```python
from build123d import *

# Parameters (mm, degrees)
SKETCH1_W           = 98
SKETCH1_H           = 98
BOSS_EXTRUDE1_DEPTH = 40
SKETCH2_W           = 94
SKETCH2_H           = 94
CUT_EXTRUDE1_DEPTH  = 5
SKETCH3_W           = 90
SKETCH3_H           = 90
CUT_EXTRUDE2_DEPTH  = 30
SKETCH4_W           = 98
SKETCH4_H           = 98
SKETCH4_W_2         = 94
SKETCH4_H_2         = 94
CUT_EXTRUDE3_DEPTH  = 1.8
SKETCH5_R           = 1.3
BOSS_EXTRUDE2_DEPTH = 2.5
FILLET1_R           = 1.5
FILLET2_R           = 1.5


with BuildPart() as part:
    # Sketch1 → Boss-Extrude1 (new body)
    with BuildSketch(Plane(origin=(0, 0, 0), x_dir=(1, 0, 0), z_dir=(0, 1, 0))):
        Rectangle(SKETCH1_W, SKETCH1_H)
    extrude(amount=BOSS_EXTRUDE1_DEPTH)

    # Sketch2 → Cut-Extrude1 (cut)
    with BuildSketch(Plane(origin=(0, 40, 0), x_dir=(1, 0, 0), z_dir=(0, 1, 0))):
        Rectangle(SKETCH2_W, SKETCH2_H)
    extrude(amount=-CUT_EXTRUDE1_DEPTH, mode=Mode.SUBTRACT)

    # Sketch3 → Cut-Extrude2 (cut)
    with BuildSketch(Plane(origin=(0, 35, 0), x_dir=(1, 0, 0), z_dir=(0, 1, 0))):
        Rectangle(SKETCH3_W, SKETCH3_H)
    extrude(amount=-CUT_EXTRUDE2_DEPTH, mode=Mode.SUBTRACT)

    # Sketch4 → Cut-Extrude3 (cut)
    with BuildSketch(Plane(origin=(0, 40, 0), x_dir=(1, 0, 0), z_dir=(0, 1, 0))):
        Rectangle(SKETCH4_W, SKETCH4_H)
        Rectangle(SKETCH4_W_2, SKETCH4_H_2, mode=Mode.SUBTRACT)
    extrude(amount=-CUT_EXTRUDE3_DEPTH, mode=Mode.SUBTRACT)

    # Sketch5 → Boss-Extrude2 (add)
    with BuildSketch(Plane(origin=(0, 38.2, 0), x_dir=(1, 0, 0), z_dir=(0, 1, 0))):
        with BuildLine():
            Line((-49, 4), (-51, 4))
            ThreePointArc((-51, 4), (-55, 0), (-51, -4))
            Line((-51, -4), (-49, -4))
            Line((-49, -4), (-49, 4))
        make_face()
        with Locations((-52.4, 0)):
            Circle(SKETCH5_R, mode=Mode.SUBTRACT)
        with BuildLine():
            Line((49, 4), (49, -4))
            Line((49, -4), (51, -4))
            ThreePointArc((51, -4), (55, 0), (51, 4))
            Line((51, 4), (49, 4))
        make_face()
        with Locations((52.4, 0)):
            Circle(SKETCH5_R, mode=Mode.SUBTRACT)
    extrude(amount=-BOSS_EXTRUDE2_DEPTH)

    # Fillet1
    fillet1_edges = [part.edges().sort_by_distance(p)[0] for p in [
        (-49, 35.7, 0),
        (-49, 36.95, -4),
        (-49, 36.95, 4),
    ]]
    fillet(fillet1_edges, radius=FILLET1_R)

    # Fillet2
    fillet2_edges = [part.edges().sort_by_distance(p)[0] for p in [
        (49, 36.95, -4),
        (49, 35.7, 0),
        (49, 36.95, 4),
    ]]
    fillet(fillet2_edges, radius=FILLET2_R)


solid = part.part
```
Part model, mm, in its own coordinate system. A direction names the side the tool comes from. Coordinates: 2 decimals unless noted, no trailing zeros. Order: outer loops, then holes, each group sorted by start corner. A loop starts at its lowest first (then second) coordinate and runs counter-clockwise, first axis right, second up. Notation, with made-up numbers: (23.5, -6) - (43.5, -6) arc R27 ccw to (43.5, 21) - close; hole circle Ø6 at (81.5, 40.5). An arc over 180 degrees is marked (long way). Return JSON: item names as keys, results as strings. Group by question number.
Item 1: Cut at D-D (z = 43). List the corners of the cut face in (x, y), plus the area to 3 significant figures.
Item 2: Which spindle directions (+Z, -Z, +X, -X, +Y, -Y) get a long thin tool onto all of the face, cutting with end or side? Do faces 1 (the face through (-1, 37, -47)), 2 (the face through (-54, 35.7, 0)), 3 (the face through (54, 35.7, 0)). Say none if no direction does.
Item 3: Cut at B-B (y = 9.5). List the corners of the cut face in (x, z), plus the area to 3 significant figures.
Item 4: Cut at A-A (z = 0). List the corners of the cut face in (x, y).
Item 5: Pin check, flat tips, straight feed: pin 1 (8 mm diameter, centred on x = -2, z = 19.5, fed in from +Y); pin 2 (1 mm diameter, centred on y = 37, z = 11.5, fed in from +X); pin 3 (1 mm diameter, centred on y = 36.5, z = -6.5, fed in from -X); pin 4 (1.3 mm diameter, centred on x = -52, z = 0, fed in from -Y). Stop position of each tip, or through.
Item 6: Cut at C-C (x = -52.4). List the corners of the cut face in (y, z), plus the area to 3 significant figures.
Item 7: Pull direction Z, two halves, no side cores. Call faces 4 (the face through (-1, 19, -49)), 5 (the face through (45, 20, 1)), 6 (the face through (-55, 37, 0)): pulls with the +Z half, pulls with the -Z half, needs draft (parallel to the pull), parting line crosses it, or undercut.
Item 8: Drill centre lines: probe 1 along X at (y, z) = (37, 0); probe 2 along Z at (x, y) = (41, 18). Where is each one in solid material? Low to high. Write a range as from..to.
Check values:
{
 "1": {"outline": "(-49, 0) - (49, 0) - (49, 38.2) - (47, 38.2) - (47, 35) - (45, 35) - (45, 5) - (-45, 5) - (-45, 35) - (-47, 35) - (-47, 38.2) - (-49, 38.2) - close", "area": "743 mm2"},
 "2": {"face 1": "+Y", "face 2": "+Z, -Z, -X, -Y", "face 3": "+Z, -Z, +X, -Y"},
 "3": {"outline": "(-49, -49) - (49, -49) - (49, 49) - (-49, 49) - close; hole (-45, -45) - (45, -45) - (45, 45) - (-45, 45) - close", "area": "1,500 mm2"},
 "4": {"outline": "(-55, 35.7) - (-53.7, 35.7) - (-53.7, 38.2) - (-55, 38.2) - close; (-51.1, 35.7) - (-50.5, 35.7) arc R1.5 cw to (-49, 34.2) - (-49, 0) - (49, 0) - (49, 34.2) arc R1.5 cw to (50.5, 35.7) - (51.1, 35.7) - (51.1, 38.2) - (47, 38.2) - (47, 35) - (45, 35) - (45, 5) - (-45, 5) - (-45, 35) - (-47, 35) - (-47, 38.2) - (-51.1, 38.2) - close; (53.7, 35.7) - (55, 35.7) - (55, 38.2) - (53.7, 38.2) - close"},
 "5": {"pin 1": "stops at y = 5", "pin 2": "stops at x = 49", "pin 3": "stops at x = -49", "pin 4": "passes through"},
 "6": {"outline": "(35.7, -3.75) - (38.2, -3.75) - (38.2, -1.3) - (35.7, -1.3) - close; (35.7, 1.3) - (38.2, 1.3) - (38.2, 3.75) - (35.7, 3.75) - close", "area": "12.2 mm2"},
 "7": {"face 4": "pulls with the -Z half", "face 5": "undercut", "face 6": "parting line crosses it"},
 "8": {"probe 1": "x = -55..-53.7, -51.1..-47, 47..51.1, 53.7..55", "probe 2": "z = -49..-45, 45..49"}
}
